Can you work these out from the model? Positions are in its coordinate system, mm. A direction names the side the tool comes from. Round coordinates to 2 decimals unless told otherwise and drop trailing zeros. Write each loop counter-clockwise with the first axis right and the second up, starting at its lowest first coordinate (ties: lowest second). Pieces come first, ordered by that corner, then holes. Notation, with made-up numbers: M 37,-2.75 L 85,-2.75 A24 ccw 85,33.25 Z; hole C -7.75,-20.75 d9. An arc over 180 degrees is marked long. Answer in a Markdown table with one row per item. Add a question column.
(1) Suppose I cut it at B-B, the plane y = 1.1. Write out the boundary of the cut face in (x, z), then the cut area to 3 significant figures.
(2) Suppose I cut it at C-C, the plane x = 11.35. Write out the boundary of the cut face in (y, z), then the cut area to 3 significant figures.
(3) I'm going to push flat-ended pins straight in: pin 1 (1.5 mm diameter, centred on y = 1.5, z = -28.5, fed in from +X); pin 2 (5 mm diameter, centred on x = -11.35, z = -9, fed in from -Y). Where does each tip first touch, or does it pass through?
(4) If I drill on probe 1 along X at (y, z) = (1.15, -9); probe 2 along Z at (x, y) = (-11.35, 0.95); probe 3 along X at (y, z) = (-0.7, -46), over which ranges is the centre line in solid material (lowest first)?
(5) Suppose I cut it at D-D, the plane z = 0. Write out the boundary of the cut face in (x, y).
(6) For faces 1 (the face through (5, 0, -36)), 2 (the face through (-5, 0, -35)), 3 (the face through (0, -1.1, -27)), which set-ups out of +Z, -Z, +X, -X, +Y, -Y let a thin tool reach every point of the face, with its end or its side?
(7) Suppose I cut it at A-A, the plane z = -9. Write out the boundary of the cut face in (x, y), then the cut area to 3 significant figures.
from build123d import *

# Parameters (mm, degrees)
ESBO_O1_R                         = 2
ESBO_O1_R_2                       = 1.5
RESSALTO_EXTRUS_O1_DEPTH          = 2
CORTE_EXTRUS_O4_REACH             = 64.33
ESBO_O4_W                         = 53
ESBO_O4_H                         = 0.9
CORTE_EXTRUS_O4_DIRECTION_2_REACH = 64.33
FILETE2_R                         = 1.5


with BuildPart() as part:
    # Esboço1 → Ressalto-extrusão1 (new, symmetric)
    with BuildSketch(Plane(origin=(0, 0, 0), x_dir=(1, 0, 0), z_dir=(0, 1, 0))):
        with BuildLine():
            Line((-13.5, 12), (-5, 12))
            Line((-5, 12), (-5, 59))
            Line((-5, 59), (5, 59))
            Line((5, 59), (5, 12))
            Line((5, 12), (13.5, 12))
            ThreePointArc((13.5, 12), (14.560660172, 11.560660172), (15, 10.5))
            Line((15, 10.5), (15, 5.746125079))
            ThreePointArc((15, 5.746125079), (14.568000959, 4.195199202), (13.396419283, 3.090938987))
            Line((13.396419283, 3.090938987), (1.62915583, -3.097717108))
            ThreePointArc((1.62915583, -3.097717108), (0, -3.5), (-1.62915583, -3.097717108))
            Line((-1.62915583, -3.097717108), (-13.396419283, 3.090938987))
            ThreePointArc((-13.396419283, 3.090938987), (-14.568000959, 4.195199202), (-15, 5.746125079))
            Line((-15, 5.746125079), (-15, 10.5))
            ThreePointArc((-15, 10.5), (-14.560660172, 11.560660172), (-13.5, 12))
        make_face()
        with Locations(Location((0, 0, 0), (0, 0, 270))):
            Circle(ESBO_O1_R, mode=Mode.SUBTRACT)
        with Locations(Location((-11.35, 9, 0), (0, 0, 270))):
            Circle(ESBO_O1_R_2, mode=Mode.SUBTRACT)
        with Locations(Location((11.35, 9, 0), (0, 0, 90))):
            Circle(ESBO_O1_R_2, mode=Mode.SUBTRACT)
    extrude(amount=RESSALTO_EXTRUS_O1_DEPTH, both=True)

    # Esboço4 → Corte-extrusão4 (cut, up to next)
    with BuildSketch(Plane.ZY.offset(5), mode=Mode.PRIVATE) as corte_extrus_o4_sk1:
        with Locations((-32.5, -1.55)):
            Rectangle(ESBO_O4_W, ESBO_O4_H)
    corte_extrus_o4_tool1 = extrude(corte_extrus_o4_sk1.sketch, amount=CORTE_EXTRUS_O4_REACH, mode=Mode.PRIVATE) & part.part
    add(corte_extrus_o4_tool1.solids().sort_by_distance((-5, -1.55, -32.5))[0], mode=Mode.SUBTRACT)

    # Esboço4 → Corte-extrusão4 direction 2 (cut, up to next)
    with BuildSketch(Plane.ZY.offset(5), mode=Mode.PRIVATE) as corte_extrus_o4_direction_2_sk1:
        with Locations((-32.5, -1.55)):
            Rectangle(ESBO_O4_W, ESBO_O4_H)
    corte_extrus_o4_direction_2_tool1 = extrude(corte_extrus_o4_direction_2_sk1.sketch, amount=-CORTE_EXTRUS_O4_DIRECTION_2_REACH, mode=Mode.PRIVATE) & part.part
    add(corte_extrus_o4_direction_2_tool1.solids().sort_by_distance((-5, -1.55, -32.5))[0], mode=Mode.SUBTRACT)

    # Filete2
    filete2_edges = [part.edges().sort_by_distance(p)[0] for p in [
        (-5, 0.45, -12),
        (-5, 0.45, -59),
        (5, 0.45, -59),
        (5, 0.45, -12),
    ]]
    fillet(filete2_edges, radius=FILETE2_R)


solid = part.part
Calculated:
| question | item | result |
|---|---|---|
| 1 | outline | M -15,-10.5 A1.5 ccw -13.5,-12 L -6.5,-12 A1.5 cw -5,-13.5 L -5,-57.5 A1.5 ccw -3.5,-59 L 3.5,-59 A1.5 ccw 5,-57.5 L 5,-13.5 A1.5 cw 6.5,-12 L 13.5,-12 A1.5 ccw 15,-10.5 L 15,-5.75 A3 ccw 13.4,-3.09 L 1.63,3.1 A3.5 ccw -1.63,3.1 L -13.4,-3.09 A3 ccw -15,-5.75 Z; hole C -11.35,-9 d3; hole C 0,0 d4; hole C 11.35,-9 d3 |
| 1 | area | 801 mm² |
| 2 | outline | M -2,-6 L -1.1,-6 L -1.1,-7.5 L 2,-7.5 L 2,-2.01 L -2,-2.01 Z; M -1.1,-12 L 2,-12 L 2,-10.5 L -1.1,-10.5 Z |
| 2 | area | 25.2 mm² |
| 3 | pin 1 | x = 5 |
| 3 | pin 2 | y = -1.1 |
| 4 | probe 1 | -15 to -12.85, -9.85 to 9.85, 12.85 to 15 |
| 4 | probe 2 | -12 to -10.5, -7.5 to -2.01 |
| 4 | probe 3 | -5 to 5 |
| 5 | outline | M -7.52,-2 L -2,-2 L -2,2 L -7.52,2 Z; M 2,-2 L 7.52,-2 L 7.52,2 L 2,2 Z |
| 6 | face 1 | -Z, +X, +Y, -Y |
| 6 | face 2 | -Z, -X, +Y, -Y |
| 6 | face 3 | -Z, +X, -X, -Y |
| 7 | outline | M -15,-1.1 L -12.85,-1.1 L -12.85,2 L -15,2 Z; M -9.85,-1.1 L 9.85,-1.1 L 9.85,2 L -9.85,2 Z; M 12.85,-1.1 L 15,-1.1 L 15,2 L 12.85,2 Z |
| 7 | area | 74.4 mm² |
